Build history of the part. All positions in model axes, mm. A direction names the side the tool comes from. Coordinates: 2 decimals unless noted, no trailing zeros. Order: outer loops, then holes, each group sorted by start corner. A loop starts at its lowest first (then second) coordinate and runs counter-clockwise, first axis right, second up. Notation, with made-up numbers: (-28.75, 2.5) -> (-9.75, 2.5) arc R4 cw to (-9.75, 9.5) -> close; hole circle Ø1 at (49, 31.25). An arc over 180 degrees is marked (long way). Write each question's results on one line, items separated by ' | '.
from build123d import *

# Parameters (mm, degrees)
EXTRUDE_1_DEPTH     = 52.5
FILLET_1_R          = 52.5
SKETCH_2_R          = 35
CUT_EXTRUDE_1_DEPTH = 105
SKETCH_3_R          = 18
EXTRUDE_2_DEPTH     = 28
RIB_1_REACH         = 193.948
SKETCH_5_WALL_W     = 459.539721034
SKETCH_5_WALL_H     = 20


with BuildPart() as part:
    # 스케치1 → 보스-돌출1 (new, symmetric)
    with BuildSketch(Plane.XY):
        Polygon((-68.904487954, -51.485249183), (-68.904487954, 4.514750817), (-15.404487954, 4.514750817), (-15.404487954, 28.514750817), (89.595512046, 28.514750817), (89.595512046, -25.485249183), (-36.731091279, -25.485249183), (-36.731091279, -51.485249183), align=None)
    extrude(amount=EXTRUDE_1_DEPTH, both=True)

    # 필렛1
    fillet_1_edges = [part.edges().sort_by_distance(p)[0] for p in [
        (-15.404487954, 16.514750817, -52.5),
        (-15.404487954, 16.514750817, 52.5),
        (89.595512046, 1.514750817, 52.5),
        (89.595512046, 1.514750817, -52.5),
    ]]
    fillet(fillet_1_edges, radius=FILLET_1_R - 0.0001)  # a hair under: the kernel refuses the full size

    # 스케치2 → 컷-돌출1 (cut)
    with BuildSketch(Plane(origin=(0, 28.514750817, 0), x_dir=(1, 0, 0), z_dir=(0, 1, 0))):
        with Locations(Location((37.095512046, 0, 0), (0, 0, 270))):
            Circle(SKETCH_2_R)
    extrude(amount=-CUT_EXTRUDE_1_DEPTH, mode=Mode.SUBTRACT)

    # 스케치3 → 보스-돌출2 (add)
    with BuildSketch(Plane.XZ.offset(51.485249183)):
        with BuildLine():
            Line((-36.731091279, 90), (-36.731091279, -90))
            ThreePointArc((-36.731091279, -90), (-76.731091279, -130), (-116.731091279, -90))
            Line((-116.731091279, -90), (-116.731091279, 90))
            ThreePointArc((-116.731091279, 90), (-76.731091279, 130), (-36.731091279, 90))
        make_face()
        with Locations(Location((-76.731091279, 90, 0), (0, 0, 270))):
            Circle(SKETCH_3_R, mode=Mode.SUBTRACT)
        with Locations(Location((-76.731091279, -90, 0), (0, 0, 270))):
            Circle(SKETCH_3_R, mode=Mode.SUBTRACT)
    extrude(amount=EXTRUDE_2_DEPTH)

    # 스케치5 wall → 보강대1 (add, up to next)
    with BuildSketch(Plane(origin=(-92.817789616, -23.485249183, 0), x_dir=(-0.649433011991, -0.76041880759, 0), z_dir=(0.76041880759, -0.649433011991, 0)), mode=Mode.PRIVATE) as rib_1_sk1:
        Rectangle(SKETCH_5_WALL_W, SKETCH_5_WALL_H)
    rib_1_tool1 = extrude(rib_1_sk1.sketch, amount=RIB_1_REACH, mode=Mode.PRIVATE) - part.part
    add(rib_1_tool1.solids().sort_by_distance((-92.817789616, -23.485249183, 0))[0])


solid = part.part
Item 1: Tool access for faces 4 (the flat face through (-82, -32, 10)), 5 (the flat face through (-68.904, -24, -31)), 6 (the flat face through (-36.731, -58, 1)): list every direction of +Z, -Z, +X, -X, +Y, -Y with a clear straight run to the whole face (end or side of a thin tool).
Answer:
face 4: +Z, -X, +Y | face 5: -Z, -X, +Y | face 6: +Z, -Z, +X, -Y
Item 2: Pull direction Z, two halves, no side cores. Call faces 1 (the cylindrical face through (2.93, 1.89, -7.59)), 2 (the flat face through (-27, -20, -52.5)), 3 (the flat face through (71, 28.515, -11)): released by +Z, released by -Z, zero draft, split by the parting line, or undercut.
Answer:
face 1: undercut | face 2: released by -Z | face 3: zero draft
Item 3: Drill centre lines: line 1 (X direction, y = -72, z = 90); line 2 (Z direction, x = -65.5, y = -58); line 3 (Y direction, x = -31.5, z = -14). Where is each one in solid material? Low to high. Write a range as from..to.
Answer:
line 1: x = -116.73..-94.73, -58.73..-36.73 | line 2: z = -128.39..-104.07, -75.93..75.93, 104.07..128.39 | line 3: y = -25.49..4.51
Item 4: Pin check, flat tips, straight feed: pin 1 (2 mm diameter, centred on y = -42.5, z = -52, fed in from -X); pin 2 (5 mm diameter, centred on y = -49, z = 4, fed in from +X); pin 3 (1 mm diameter, centred on x = -69.5, y = -68.5, fed in from +Z). Stop position of each tip, or through.
Answer:
pin 1: stops at x = -68.9 | pin 2: stops at x = -36.73 | pin 3: stops at z = 129.43
Item 5: Slice it at B-B, the plane z = -99. List the corners of the cut face in (x, y), and give its area (3 significant figures).
Answer:
outline: (-115.71, -79.49) -> (-92.32, -79.49) -> (-92.32, -51.49) -> (-115.71, -51.49) -> close; (-61.14, -79.49) -> (-37.76, -79.49) -> (-37.76, -51.49) -> (-61.14, -51.49) -> close | area: 1,310 mm^2
Item 6: Slice it at A-A, the plane x = -64. List the corners of the cut face in (y, z), and give its area (3 significant figures).
Answer:
outline: (-79.49, -127.92) -> (-51.49, -127.92) -> (-51.49, -102.72) -> (-79.49, -102.72) -> close; (-79.49, -77.28) -> (-51.49, -77.28) -> (-51.49, -52.5) -> (4.51, -52.5) -> (4.51, 52.5) -> (-51.49, 52.5) -> (-51.49, 77.28) -> (-79.49, 77.28) -> close; (-79.49, 102.72) -> (-51.49, 102.72) -> (-51.49, 127.92) -> (-79.49, 127.92) -> close | area: 11,600 mm^2
Item 7: Slice it at D-D, the plane y = -34.5. List the corners of the cut face in (x, z), and give its area (3 significant figures).
Answer:
outline: (-102.22, -10) -> (-68.9, -10) -> (-68.9, -52.5) -> (-36.73, -52.5) -> (-36.73, 52.5) -> (-68.9, 52.5) -> (-68.9, 10) -> (-102.22, 10) -> close | area: 4,040 mm^2
Item 8: Slice it at C-C, the plane x = 19. List the corners of the cut face in (y, z), and give its area (3 significant figures).
Answer:
outline: (-25.49, -52.5) -> (4.51, -52.5) -> (4.51, -49.28) -> (28.51, -49.28) -> (28.51, -29.96) -> (-25.49, -29.96) -> close; (-25.49, 29.96) -> (28.51, 29.96) -> (28.51, 49.28) -> (4.51, 49.28) -> (4.51, 52.5) -> (-25.49, 52.5) -> close | area: 2,280 mm^2
